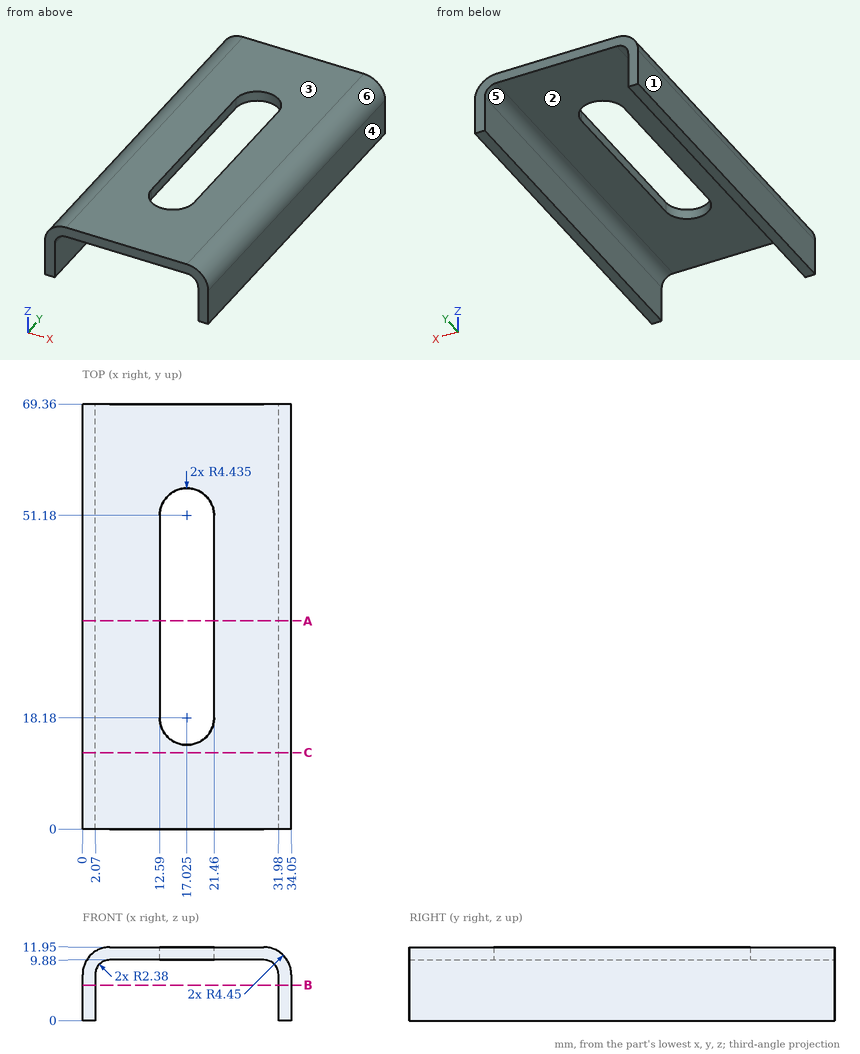
Here's the drawing with two shaded views (mm, measured from the low corner). I have some questions. A direction names the side the tool comes from. Round coordinates to 2 decimals unless told otherwise and drop trailing zeros. Loops run counter-clockwise (first coordinate to the right, second up) from the corner with the lowest first, then second, coordinate; pieces in that order, holes last. Notation, with made-up numbers: (-22, 55.5) -> (-4, 55.5) arc R27 ccw to (-4, 74.5) -> close; hole circle Ø1 at (-1.5, 5.5). An arc over 180 degrees is marked (long way). Answer as CSV lines item,"result". Start each with the question number.
1. Imagine slicing it at A-A on y = 34. Write out the boundary of the cut face in (x, z).
2. I'm going to push flat-ended pins straight in: P1, Ø4, axis at x = 17.5, z = 6, coming from the +Y side; P2, Ø0.6, axis at y = 29, z = 11, coming from the +X side; P3, Ø1, axis at y = 28.5, z = 10.5, coming from the -X side; P4, Ø7.5, axis at x = 19.5, y = 18.5, coming from the -Z side. Where does each tip first touch, or does it pass through?
3. Imagine slicing it at C-C on y = 12.5. Write out the boundary of the cut face in (x, z).
4. I need wall thicknesses on probe 1 along X at (y, z) = (32.5, 2); probe 2 along X at (y, z) = (26.5, 8.5); probe 3 along Z at (x, y) = (11.5, 52.5). Which ranges of each line are inside material? Lowest first, please. Write a range as from..to.
5. For the marked faces 5 and 6, which set-ups out of +Z, -Z, +X, -X, +Y, -Y let a thin tool reach every point of the face, with its end or its side?
6. Imagine slicing it at B-B on z = 5.75. Write out the boundary of the cut face in (x, y), plus the area to 3 significant figures.
7. If we mould it in two halves opening along X, with no side actions, what happens to the marked faces 1, 2, 3 and 4? For each: pulls with the +X half, pulls with the -X half, needs draft (parallel to the pull), parting line crosses it, or undercut.
Solution:
1,outline,"(0, 0) -> (2.07, 0) -> (2.07, 7.5) arc R2.38 cw to (4.45, 9.88) -> (12.59, 9.88) -> (12.59, 11.95) -> (4.45, 11.95) arc R4.45 ccw to (0, 7.5) -> close; (21.46, 9.88) -> (29.6, 9.88) arc R2.38 cw to (31.98, 7.5) -> (31.98, 0) -> (34.05, 0) -> (34.05, 7.5) arc R4.45 ccw to (29.6, 11.95) -> (21.46, 11.95) -> close"
2,P1,"through"
2,P2,"x = 32.69"
2,P3,"x = 0.77"
2,P4,"z = 9.88"
3,outline,"(0, 0) -> (2.07, 0) -> (2.07, 7.5) arc R2.38 cw to (4.45, 9.88) -> (29.6, 9.88) arc R2.38 cw to (31.98, 7.5) -> (31.98, 0) -> (34.05, 0) -> (34.05, 7.5) arc R4.45 ccw to (29.6, 11.95) -> (4.45, 11.95) arc R4.45 ccw to (0, 7.5) -> close"
4,probe 1,"0..2.07, 31.98..34.05"
4,probe 2,"0.11..2.29, 31.76..33.94"
4,probe 3,"9.88..11.95"
5,face 5,"-Z, +Y, -Y"
5,face 6,"+Z, +X, +Y, -Y"
6,outline,"(0, 0) -> (2.07, 0) -> (2.07, 69.36) -> (0, 69.36) -> close; (31.98, 0) -> (34.05, 0) -> (34.05, 69.36) -> (31.98, 69.36) -> close"
6,area,"287 mm²"
7,face 1,"pulls with the -X half"
7,face 2,"undercut"
7,face 3,"needs draft"
7,face 4,"pulls with the +X half"
